Answer from the drawing. Dimensions are ordinates in mm from the lowest x, y and z of the part. Round coordinates to 2 decimals unless told otherwise and drop trailing zeros. Loops run counter-clockwise (first coordinate to the right, second up) from the corner with the lowest first, then second, coordinate; pieces in that order, holes last. Notation, with made-up numbers: (-38, 75.5) - (-22, 75.5) arc R26 ccw to (-22, 107.5) - close; hole circle Ø10 at (65, 87). An arc over 180 degrees is marked (long way). Answer as CSV lines item,"result".
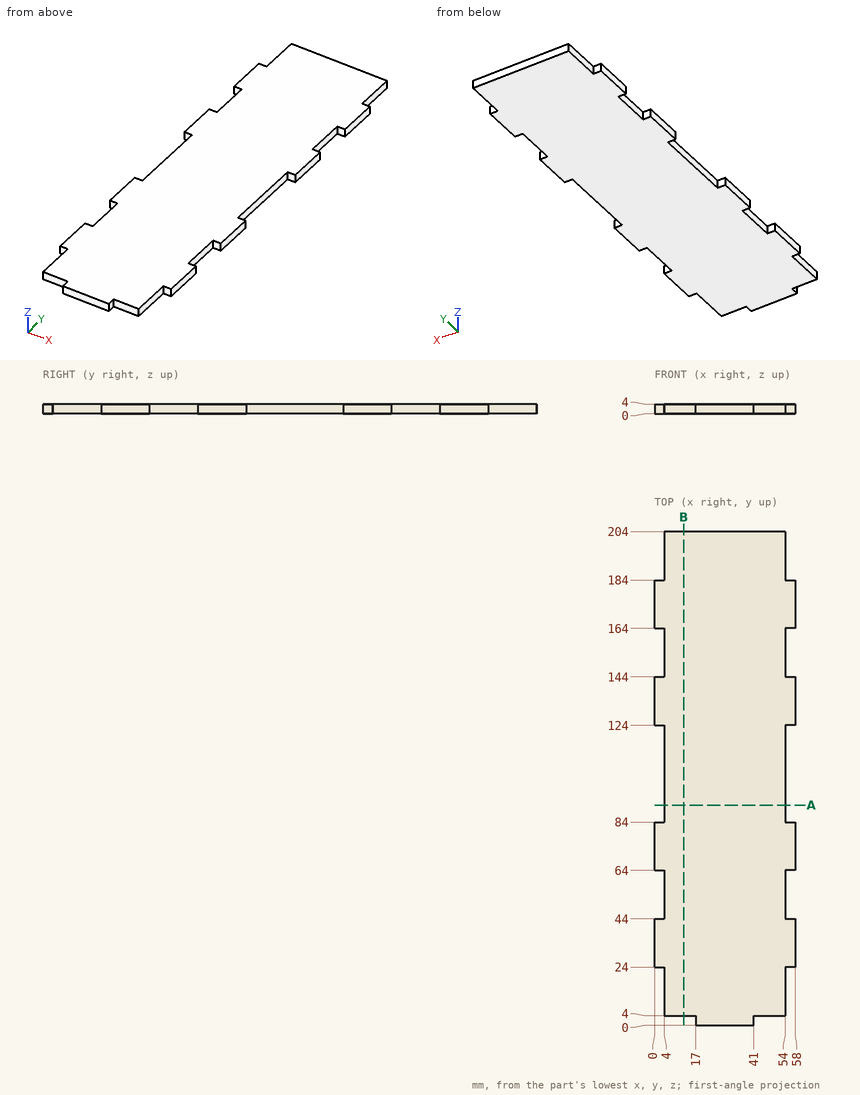
1) Each of these flat-tipped pins is pushed along its axis until it touches: P1, Ø1.2, axis at y = 15.5, z = 1.5, coming from the +X side; P2, Ø2, axis at x = 1.5, z = 3, coming from the -Y side; P3, Ø2, axis at y = 17, z = 2.5, coming from the -X side. Where does it stop, or does it pass through?
Entries:
P1,"stops at x = 54"
P2,"stops at y = 24"
P3,"stops at x = 4"
2) A cutting plane is placed at B-B, the plane x = 12. Determine the outline of the cut face in (y, z), plus the area to 3 significant figures.
Entries:
outline,"(4, 0) - (204, 0) - (204, 4) - (4, 4) - close"
area,"800 mm^2"
3) Find the intervals of material crossed by line 1 (Y direction, x = 55.5, z = 0.5); line 2 (X direction, y = 194.5, z = 0.6); line 3 (Y direction, x = 10, z = 2.6), in increasing order.
Entries:
line 1,"y = 24 to 44, 64 to 84, 124 to 144, 164 to 184"
line 2,"x = 4 to 54"
line 3,"y = 4 to 204"
4) A cutting plane is placed at A-A, the plane y = 91. Determine the outline of the cut face in (x, z), plus the area to 3 significant figures.
Entries:
outline,"(4, 0) - (54, 0) - (54, 4) - (4, 4) - close"
area,"200 mm^2"
